Can you work these out from the model? Positions are in its coordinate system, mm. Face numbers are marked on the shaded views. Give positions to 0.01 mm unless a question says otherwise; leave off trailing zeros. Write each loop counter-clockwise with the first axis right and the second up, starting at its lowest first coordinate (ties: lowest second). Pieces come first, ordered by that corner, then holes. Notation, with made-up numbers: M 79.25,30.5 L 128.25,30.5 A26 ccw 128.25,69.5 Z; hole C 56,85.25 d4. An arc over 180 degrees is marked long. Write each question's results on one line, items separated by ' | '.
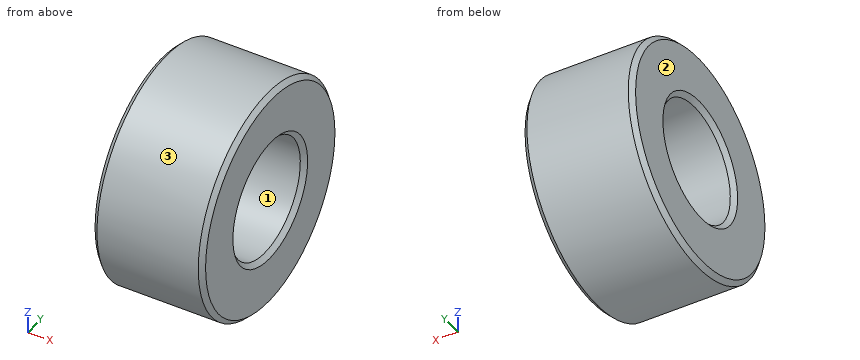
from build123d import *

# Parameters (mm, degrees)
SKETCH1_W     = 6
SKETCH1_H     = 3
CHAMFER1_SIZE = 0.25


with BuildPart() as part:
    # Sketch1 → Revolve1 (revolve)
    with BuildSketch(Plane.XY, mode=Mode.PRIVATE) as revolve1_sk:
        with Locations((0, 4.675)):
            Rectangle(SKETCH1_W, SKETCH1_H)
    revolve(revolve1_sk.sketch.rotate(Axis((0, 0, 0), (1, 0, 0)), 90), axis=Axis((0, 0, 0), (1, 0, 0)))

    # Chamfer1
    chamfer1_edges = [part.edges().sort_by_distance(p)[0] for p in [
        (-3, 0, -3.175),
        (3, 0, -3.175),
        (3, 0, -6.175),
        (-3, 0, -6.175),
    ]]
    chamfer(chamfer1_edges, length=CHAMFER1_SIZE)


solid = part.part
Item 1: If I drill on line 1 (Y direction, x = 0.4, z = 0) (3 decimals); line 2 (Z direction, x = -1.35, y = -1.75); line 3 (Y direction, x = 0.8, z = -2), over which ranges is the centre line in solid material (lowest first)? Write a range as from..to.
Geometry says:
line 1: y = -6.175..-3.175, 3.175..6.175 | line 2: z = -5.92..-2.65, 2.65..5.92 | line 3: y = -5.84..-2.47, 2.47..5.84
Item 2: I'm going to push flat-ended pins straight in: pin 1 (2 mm diameter, centred on x = -2, y = -3.5, fed in from -Z); pin 2 (5.5 mm diameter, centred on y = 0, z = 0, fed in from +X); pin 3 (1 mm diameter, centred on x = -0.5, y = 5, fed in from -Z). Where does each tip first touch, or does it pass through?
Geometry says:
pin 1: stops at z = -5.65 | pin 2: passes through | pin 3: stops at z = -4.23
Item 3: I want a section at C-C, the plane x = -2.4. Please give me the cut outline in (y, z) (3 decimals), and give its area (3 significant figures).
Geometry says:
outline: C 0,0 d12.35; hole C 0,0 d6.35 | area: 88.1 mm2
Item 4: I want a section at A-A, the plane y = 0. Please give me the cut outline in (x, z) (3 decimals).
Geometry says:
outline: M -3,-5.925 L -2.75,-6.175 L 2.75,-6.175 L 3,-5.925 L 3,-3.425 L 2.75,-3.175 L -2.75,-3.175 L -3,-3.425 Z; M -3,3.425 L -2.75,3.175 L 2.75,3.175 L 3,3.425 L 3,5.925 L 2.75,6.175 L -2.75,6.175 L -3,5.925 Z
Item 5: Thinking about a two-plate mould opening in Z: for the marked faces 1, 2 and 3, which applies, +Z half, -Z half, draft (parallel to the pull), parting line (faces both ways), or undercut?
Geometry says:
face 1: undercut | face 2: draft | face 3: parting line
